Part model, mm, in its own coordinate system. Face numbers are marked on the shaded views. Round coordinates to 2 decimals unless told otherwise and drop trailing zeros. Loops run counter-clockwise (first coordinate to the right, second up) from the corner with the lowest first, then second, coordinate; pieces in that order, holes last.
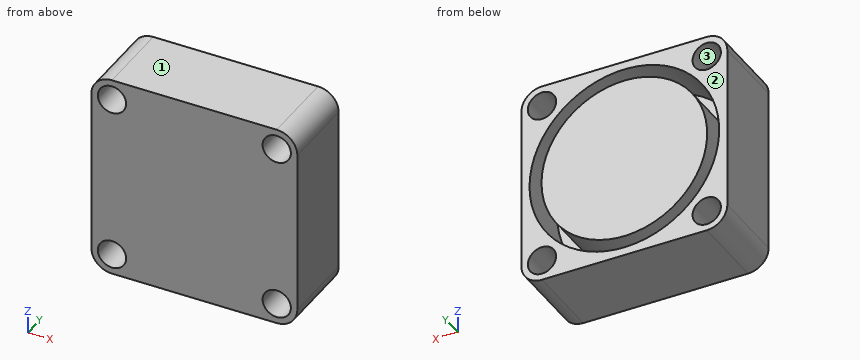
Autodesk Inventor part; units mm, degrees
ref_plane "YZ Plane" through (0, 0, 0) normal (1, 0, 0) x (0, 1, 0)
ref_plane "XZ Plane" through (0, 0, 0) normal (0, 1, 0) x (-1, 0, 0)
ref_plane "XY Plane" through (0, 0, 0) normal (0, 0, 1) x (1, 0, 0)
sketch "Sketch1" plane through (0, 0, 0) normal (0, 1, 0) x (-1, 0, 0)
  line L0 (16, 20) -> (-16, 20)
  line L1 (-20, 16) -> (-20, -16)
  line L2 (-16, -20) -> (16, -20)
  line L3 (20, -16) -> (20, 16)
  arc A0 (16, -20) -> (20, -16) centre (16, -16) ccw
  arc A1 (-20, -16) -> (-16, -20) centre (-16, -16) ccw
  arc A2 (20, 16) -> (16, 20) centre (16, 16) ccw
  arc A3 (-16, 20) -> (-20, 16) centre (-16, 16) ccw
  circle A4 centre (16, -16) radius 2.75
  circle A5 centre (-16, -16) radius 2.75
  circle A6 centre (16, 16) radius 2.75
  circle A7 centre (-16, 16) radius 2.75
  point P0 (0, 0)
  point P1 (-20, -20)
  point P2 (20, -20)
  point P3 (0, -20)
  point P4 (20, 0)
  dimension "d1" = 40
  dimension "d17" = 5.5
  dimension "d22" = 32
extrude "Extrusion1" add sketch "Sketch1" along normal blind 15
sketch "Sketch2" plane through (0, 15, 0) normal (0, 1, 0) x (1, 0, 0)
  circle A0 centre (0, 0) radius 18.4191
  circle A1 centre (0, 0) radius 16.0895
extrude "Extrusion2" cut sketch "Sketch2" against normal blind 10
properties part number "Fan" material "ABS Plastic"
1) Slice it at C-C, the plane x = 0. Give the cut face in (y, z).
Values:
outline: (0, -20) - (15, -20) - (15, -18.42) - (5, -18.42) - (5, -16.09) - (15, -16.09) - (15, 16.09) - (5, 16.09) - (5, 18.42) - (15, 18.42) - (15, 20) - (0, 20) - close
2) Mould opens along Z. For the marked faces 1, 2 and 3 say: released by +Z, released by -Z, zero draft, split by the parting line, or undercut.
Values:
face 1: released by +Z
face 2: zero draft
face 3: undercut
3) Slice it at B-B, the plane y = 4.25. Give the cut face in (x, z).
Values:
outline: (-20, -16) arc R4 ccw to (-16, -20) - (16, -20) arc R4 ccw to (20, -16) - (20, 16) arc R4 ccw to (16, 20) - (-16, 20) arc R4 ccw to (-20, 16) - close; hole circle Ø5.5 at (-16, -16); hole circle Ø5.5 at (-16, 16); hole circle Ø5.5 at (16, -16); hole circle Ø5.5 at (16, 16)
4) Slice it at A-A, the plane y = 9. Give the cut face in (x, z), then the cut area to 3 significant figures.
Values:
outline: (-20, -16) arc R4 ccw to (-16, -20) - (16, -20) arc R4 ccw to (20, -16) - (20, 16) arc R4 ccw to (16, 20) - (-16, 20) arc R4 ccw to (-20, 16) - close; circle Ø32.18 at (0, 0); hole circle Ø5.5 at (-16, -16); hole circle Ø5.5 at (-16, 16); hole circle Ø36.84 at (0, 0); hole circle Ø5.5 at (16, -16); hole circle Ø5.5 at (16, 16)
area: 1,240 mm2
5) Slice it at D-D, the plane z = 0. Give the cut face in (x, y), then the cut area to 3 significant figures.
Values:
outline: (-20, 0) - (20, 0) - (20, 15) - (18.42, 15) - (18.42, 5) - (16.09, 5) - (16.09, 15) - (-16.09, 15) - (-16.09, 5) - (-18.42, 5) - (-18.42, 15) - (-20, 15) - close
area: 553 mm2
6) Wall check: line 1 along Z through (x, y) = (0, 9); line 2 along Z through (x, y) = (-16, 4.25). Give the ranges that are in metal, low to high.
Values:
line 1: z = -20 to -18.42, -16.09 to 16.09, 18.42 to 20
line 2: z = -20 to -18.75, -13.25 to 13.25, 18.75 to 20
